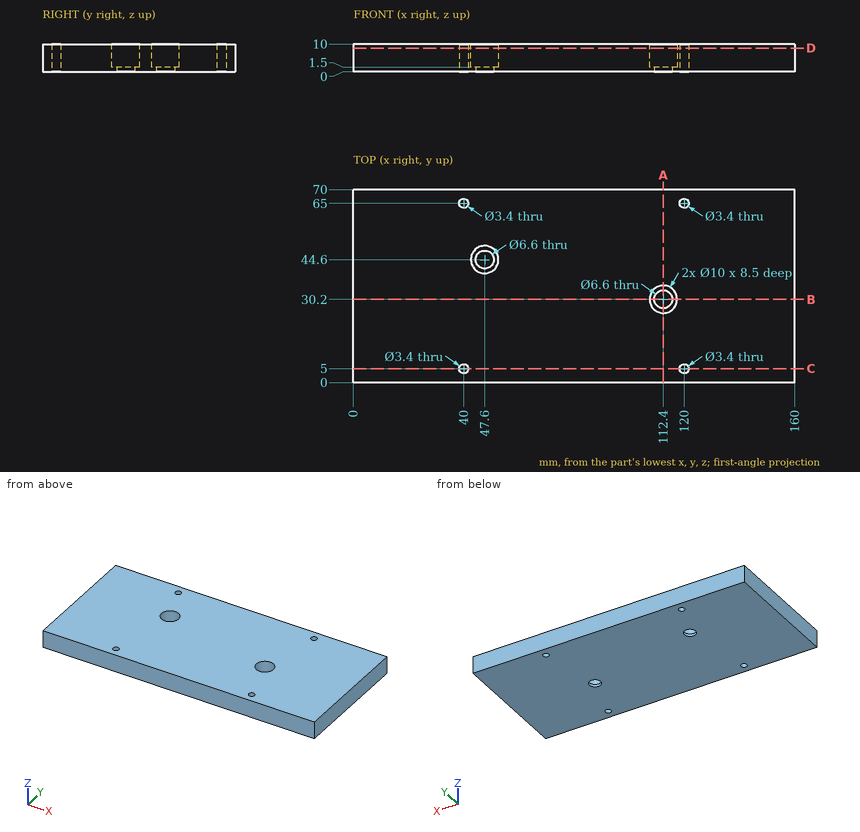
Geometry check sheet. Reference: drawing and pictorial views, mm from the part's lowest x, y, z. Round coordinates to 2 decimals unless told otherwise and drop trailing zeros. Order: outer loops, then holes, each group sorted by start corner. A loop starts at its lowest first (then second) coordinate and runs counter-clockwise, first axis right, second up.
Q1. Scan lines: L1, parallel to Y at x = 40, z = 5.75; L2, parallel to X at y = 65, z = 6; L3, parallel to Y at x = 112.4, z = 7.75. Record each from-to range of solid material in increasing order.
Filled sheet:
L1: y = 0 to 3.3, 6.7 to 63.3, 66.7 to 70
L2: x = 0 to 38.3, 41.7 to 118.3, 121.7 to 160
L3: y = 0 to 25.2, 35.2 to 70
Q2. Cross-section at D-D, the plane z = 8.5. Enter the section's corners in (x, y).
Filled sheet:
outline: (0, 0) - (160, 0) - (160, 70) - (0, 70) - close; hole circle Ø3.4 at (40, 5); hole circle Ø3.4 at (40, 65); hole circle Ø10 at (47.6, 44.6); hole circle Ø10 at (112.4, 30.2); hole circle Ø3.4 at (120, 5); hole circle Ø3.4 at (120, 65)
Q3. Cross-section at A-A, the plane x = 112.4. Enter the section's corners in (y, z).
Filled sheet:
outline: (0, 0) - (26.9, 0) - (26.9, 1.5) - (25.2, 1.5) - (25.2, 10) - (0, 10) - close; (33.5, 0) - (70, 0) - (70, 10) - (35.2, 10) - (35.2, 1.5) - (33.5, 1.5) - close
Q4. Cross-section at C-C, the plane y = 5. Enter the section's corners in (x, z), plus the area to 3 significant figures.
Filled sheet:
outline: (0, 0) - (38.3, 0) - (38.3, 10) - (0, 10) - close; (41.7, 0) - (118.3, 0) - (118.3, 10) - (41.7, 10) - close; (121.7, 0) - (160, 0) - (160, 10) - (121.7, 10) - close
area: 1,530 mm2
Q5. Depth check by flat-ended pin: P1, Ø4, axis at x = 120, y = 5, coming from the +Z side; P2, Ø6, axis at x = 47.6, y = 44.6, coming from the +Z side; P3, Ø8, axis at x = 112.4, y = 30.2, coming from the +Z side. Enter the tip coordinate at first touch or a pass-through.
Filled sheet:
P1: stops at z = 10
P2: passes through
P3: stops at z = 1.5
Q6. Cross-section at B-B, the plane y = 30.2. Enter the section's corners in (x, z), plus the area to 3 significant figures.
Filled sheet:
outline: (0, 0) - (109.1, 0) - (109.1, 1.5) - (107.4, 1.5) - (107.4, 10) - (0, 10) - close; (115.7, 0) - (160, 0) - (160, 10) - (117.4, 10) - (117.4, 1.5) - (115.7, 1.5) - close
area: 1,510 mm2
